Autodesk Fusion 360 part; units mm, degrees
sketch "Z motor reinforcement" plane through (0, 0, 0) normal (0, 1, 0) x (1, 0, 0)
  line L0 (-70, -17.4987) -> (70, -17.4987)
  circle A0 centre (-45, -11.9987) radius 3
  circle A1 centre (-45, 12.0013) radius 3
  circle A2 centre (45, -11.9987) radius 3
  circle A3 centre (45, 12.0013) radius 3
  circle A4 centre (20, -11.9799) radius 2.5
  line L1 (45, -13.5) -> (45, 16.5) construction
  line L2 (20, -13.5) -> (20, 16.5) construction
  line L3 (-54.8652, -11.9987) -> (55.1348, -11.9987) construction
  line L4 (70, 17.5013) -> (-70, 17.5013)
  line L5 (-45, -13.5) -> (-45, 16.5) construction
  line L6 (70, -17.4987) -> (70, 17.5013)
  line L7 (20, -11.9799) -> (20, 12) construction
  circle A5 centre (20, 12) radius 2.5
  line L8 (-55, 12.0013) -> (55, 12.0013) construction
  circle A6 centre (-20, 12) radius 2.5
  line L9 (-70, 17.5013) -> (-70, -17.4987)
  line L10 (-20, -11.985) -> (-20, 12) construction
  line L11 (-20, -13.5) -> (-20, 16.5) construction
  circle A7 centre (-20, -11.985) radius 2.5
  dimension "d1" = 140
  dimension "d2" = 35
  dimension "d3" = 110
  dimension "d4" = 24
  dimension "d5" = 25
  dimension "d6" = 40
  dimension "d7" = 25
  dimension "d8" = 25
  dimension "d9" = 6
  dimension "d10" = 6
  dimension "d11" = 6
  dimension "d12" = 6
  dimension "d13" = 5
  dimension "d14" = 5
  dimension "d15" = 5
  dimension "d16" = 5
  dimension "d17" = 5.5
extrude "Extrude1" add sketch "Z motor reinforcement" along normal blind 6 makes body 1
copy_body "Body->Comp1" bodies 1 removing the originals makes body 2 in component "Z motor reinforcement"
chamfer "Chamfer1" distance 0.5 angle 45 27 edges at (0, 0, 17.4987) (-70, 3, 17.4987) (0, 6, 17.4987) (70, 3, 17.4987) (70, 6, -0.0013) (70, 0, -0.0013) (0, 0, -17.5013) (-70, 0, -0.0013) (-47.797, 0, 10.9138) (-47.797, 0, -13.0862) (-22.3308, 0, 11.081) (-22.3308, 0, -12.904) (17.6692, 0, 11.0759) (17.6692, 0, -12.904) (42.203, 0, 10.9138) (42.203, 0, -13.0862) (0, 6, -17.5013) (-70, 3, -17.5013) (-70, 6, -0.0013) (-47.797, 6, -13.0862) (-47.797, 6, 10.9138) (-22.3308, 6, 11.081) (17.6692, 6, 11.0759) (42.203, 6, 10.9138) (42.203, 6, -13.0862) (17.6692, 6, -12.904) (-22.3308, 6, -12.904) on bodies 2 in component "Z motor reinforcement"
component "Z motor reinforcement" placed x (1, 0, 0) y (0, 1, 0) z (0, 0, 1) at (0, 0, 0)
Input: part model. Units: mm. Frame: model coordinates. Give positions to 0.01 mm unless a question says otherwise; leave off trailing zeros. Loops run counter-clockwise (first coordinate to the right, second up) from the corner with the lowest first, then second, coordinate; pieces in that order, holes last.
1) Contact query for a flat-ended pin moving along its axis: pin 1 (4 mm diameter, centred on x = -20, z = 11.985, fed in from +Y). Output: stop coordinate, or through.
A:
pin 1: passes through
2) Mould query, pull axis X, two halves, no side actions, for faces 1 (the cylindrical face through (-22, 3, -13.5)), 2 (the flat face through (1, 3, -17.501)), 3 (the flat face through (-70, 3, 0)). Classes: released by +X, released by -X, zero draft, split by the parting line, or undercut.
A:
face 1: undercut
face 2: zero draft
face 3: released by -X
3) Section query C-C on x = -20. Return the cut outline in (y, z) (3 decimals), and give its area (4 significant figures).
A:
outline: (0, -17.001) - (0.5, -17.501) - (5.5, -17.501) - (6, -17.001) - (6, -15) - (5.5, -14.5) - (0.5, -14.5) - (0, -15) - close; (0, -9) - (0.5, -9.5) - (5.5, -9.5) - (6, -9) - (6, 8.985) - (5.5, 9.485) - (0.5, 9.485) - (0, 8.985) - close; (0, 14.985) - (0.5, 14.485) - (5.5, 14.485) - (6, 14.985) - (6, 16.999) - (5.5, 17.499) - (0.5, 17.499) - (0, 16.999) - close
area: 148.5 mm2
4) Section query A-A on x = -45. Return the cut outline in (y, z), and give its area (4 significant figures).
A:
outline: (0, -17) - (0.5, -17.5) - (5.5, -17.5) - (6, -17) - (6, -15.5) - (5.5, -15) - (0.5, -15) - (0, -15.5) - close; (0, -8.5) - (0.5, -9) - (5.5, -9) - (6, -8.5) - (6, 8.5) - (5.5, 9) - (0.5, 9) - (0, 8.5) - close; (0, 15.5) - (0.5, 15) - (5.5, 15) - (6, 15.5) - (6, 17) - (5.5, 17.5) - (0.5, 17.5) - (0, 17) - close
area: 136.5 mm2
5) Section query B-B on y = 4.25. Count the separate pieces of the cut face and the enclosed holes in it, and give its area (3 significant figures).
A:
separate pieces: 1
enclosed holes: 8
area: 4,710 mm2
6) Line query: L1, parallel to Z at x = 45, y = 2.3; L2, parallel to Z at x = 20, y = 1.9; L3, parallel to X at y = 2.85, z = -12. Output: solid intervals per line, ascending.
A:
L1: z = -17.5 to -15, -9 to 9, 15 to 17.5
L2: z = -17.5 to -14.5, -9.5 to 9.48, 14.48 to 17.5
L3: x = -70 to -48, -42 to -22.5, -17.5 to 17.5, 22.5 to 42, 48 to 70
